Geometry: final body of the model. Coordinates: model frame, mm. Coordinates: 2 decimals unless noted, no trailing zeros. Order: outer loops, then holes, each group sorted by start corner. A loop starts at its lowest first (then second) coordinate and runs counter-clockwise, first axis right, second up. Notation, with made-up numbers: M -1,25 L 21,25 A30 cw 21,63 Z; hole C 77,-19 d7. An arc over 180 degrees is marked long. Use CSV: the item, a comma, the result in double quotes. Start each with the question number.
Q1. Section query A-A, the plane y = 2.5. Output: boundary loops of the cut face in (x, z).
Q2. Section query B-B, the plane z = 55. Output: boundary loops of the cut face in (x, y), and give its area (3 significant figures).
Q3. Section query D-D, the plane z = -28. Output: boundary loops of the cut face in (x, y), and give its area (3 significant figures).
Q4. Ray query, probe 1 along Z at (x, y) = (55, 5); probe 2 along X at (y, z) = (0.5, -50.5). Return the intervals inside material, ascending.
Q5. Section query C-C, the plane x = 55. Output: boundary loops of the cut face in (y, z), and give its area (3 significant figures).
Q6. First-contact query: P1, Ø3, axis at y = 4.5, z = 64, coming from the -X side; P2, Ø4, axis at x = -43, y = 5, coming from the -Z side. Flat tips, straight axial feed; report the tip coordinate or a pass-through.
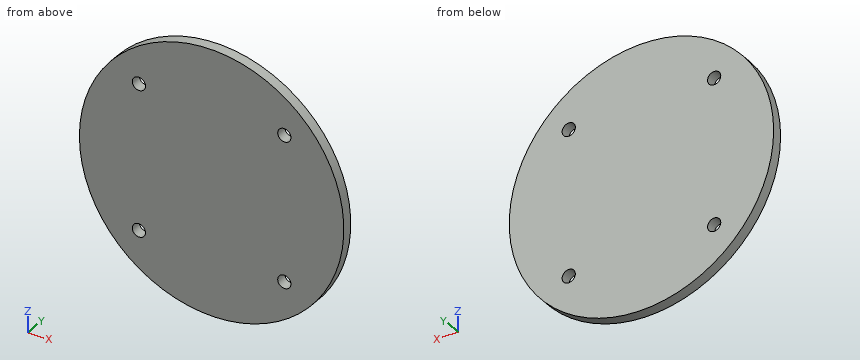
Autodesk Inventor part; units mm, degrees
ref_plane "YZ Plane" through (0, 0, 0) normal (1, 0, 0) x (0, 1, 0)
ref_plane "XZ Plane" through (0, 0, 0) normal (0, 1, 0) x (-1, 0, 0)
ref_plane "XY Plane" through (0, 0, 0) normal (0, 0, 1) x (1, 0, 0)
sketch "Esquisse1" plane through (0, 0, 0) normal (0, 1, 0) x (-1, 0, 0)
  circle A0 centre (0, 0) radius 100
  line L0 (55, -55) -> (-55, -55)
  line L1 (-55, -55) -> (-55, 55)
  line L2 (-55, 55) -> (55, 55)
  line L3 (55, 55) -> (55, -55)
  line L4 (55, -55) -> (-55, 55) construction
  line L5 (-55, -55) -> (55, 55) construction
  circle A1 centre (-55, 55) radius 5
  circle A2 centre (55, 55) radius 5
  circle A3 centre (55, -55) radius 5
  circle A4 centre (-55, -55) radius 5
  dimension "d0" = 200
  dimension "d3" = 110
  dimension "d4" = 10
extrude "Extrusion1" add sketch "Esquisse1" along normal blind 8 contours A0 | A4 L1 L0 | A4 L1 A1 L2 A2 L3 A3 L0 | L0 L1 A4 | A3 L3 L0 | L0 L3 A3 | A1 L2 L1 | L1 L2 A1 | A2 L2 L3 | L3 L2 A2
sketch "Esquisse2" plane through (0, 0, 0) normal (0, -1, 0) x (1, 0, 0)
  line L0 (-55, -55) -> (55, -55)
  line L1 (55, -55) -> (55, 55)
  line L2 (55, 55) -> (-55, 55)
  line L3 (-55, 55) -> (-55, -55)
  line L4 (-55, -55) -> (55, 55) construction
  line L5 (55, -55) -> (-55, 55) construction
  circle A0 centre (-55, 55) radius 5
  circle A1 centre (55, 55) radius 5
  circle A2 centre (55, -55) radius 5
  circle A3 centre (-55, -55) radius 5
  point P0 (0, 0)
  dimension "d5" = 110
  dimension "d6" = 10
extrude "Extrusion2" cut sketch "Esquisse2" against normal blind 10 contours L3 A3 L0 | L0 A3 L3 | A2 L1 L0 | L0 L1 A2 | A0 L2 L3 | L3 L2 A0 | A1 L2 L1 | L1 L2 A1
properties part number "base" material "Bois (bouleau)"
Responses:
1,outline,"C 0,0 d200; hole C -55,-55 d10; hole C -55,55 d10; hole C 55,-55 d10; hole C 55,55 d10"
2,outline,"M -83.52,0 L -60,0 L -60,8 L -83.52,8 Z; M -50,0 L 50,0 L 50,8 L -50,8 Z; M 60,0 L 83.52,0 L 83.52,8 L 60,8 Z"
2,area,"1,180 mm²"
3,outline,"M -96,0 L 96,0 L 96,8 L -96,8 Z"
3,area,"1,540 mm²"
4,probe 1,"z = -83.52 to -60, -50 to 50, 60 to 83.52"
4,probe 2,"x = -86.31 to -57.18, -52.82 to 52.82, 57.18 to 86.31"
5,outline,"M 0,-83.52 L 8,-83.52 L 8,-60 L 0,-60 Z; M 0,-50 L 8,-50 L 8,50 L 0,50 Z; M 0,60 L 8,60 L 8,83.52 L 0,83.52 Z"
5,area,"1,180 mm²"
6,P1,"stops at x = -78.06"
6,P2,"stops at z = -91.21"
